```python
from build123d import *

# Parameters (mm, degrees)
PAD_DEPTH    = 1.56
PAD001_DEPTH = 1.56
SKETCH002_W  = 11.4
SKETCH002_H  = 3.36
PAD002_DEPTH = 0.1
SKETCH003_W  = 11.4
SKETCH003_H  = 0.1
PAD003_DEPTH = 9.6
FILLET_R     = 1
FILLET001_R  = 1
POCKET_DEPTH = 0.2


with BuildPart() as part:
    # Sketch → Pad (new body)
    with BuildSketch(Plane.XY):
        with BuildLine():
            Line((-9.985, 17.165), (9.985, 17.165))
            ThreePointArc((13.985, 13.165), (12.813427, 15.993427), (9.985, 17.165))
            Line((13.985, 13.165), (13.985, -13.165))
            ThreePointArc((9.985, -17.165), (12.813427, -15.993427), (13.985, -13.165))
            Line((9.985, -17.165), (-9.985, -17.165))
            ThreePointArc((-13.985, -13.165), (-12.813427, -15.993427), (-9.985, -17.165))
            Line((-13.985, -13.165), (-13.985, 13.165))
            ThreePointArc((-9.985, 17.165), (-12.813427, 15.993427), (-13.985, 13.165))
        make_face()
    extrude(amount=PAD_DEPTH)

    # Sketch001 (on Face10 of Pad) → Pad001 (join)
    with BuildSketch(Plane.XY.offset(1.56)):
        with BuildLine():
            Line((-10.035, 18.165), (10.035, 18.165))
            ThreePointArc((15.035, 13.165), (13.570534, 16.700534), (10.035, 18.165))
            Line((15.035, 13.165), (15.035, -14.264405))
            ThreePointArc((10.035, -19.264405), (13.570534, -17.799939), (15.035, -14.264405))
            Line((10.035, -19.264405), (-10.035, -19.264405))
            ThreePointArc((-15.035, -14.264405), (-13.570534, -17.799939), (-10.035, -19.264405))
            Line((-15.035, -14.264405), (-15.035, 13.165))
            ThreePointArc((-10.035, 18.165), (-13.570534, 16.700534), (-15.035, 13.165))
        make_face()
    extrude(amount=-PAD001_DEPTH)

    # Sketch002 (on Face10 of Pad001) → Pad002 (join)
    with BuildSketch(Plane.XZ.offset(19.264405)):
        with Locations((0, 1.68)):
            Rectangle(SKETCH002_W, SKETCH002_H)
    extrude(amount=PAD002_DEPTH)

    # Sketch003 (on Face11 of Pad002) → Pad003 (join)
    with BuildSketch(Plane(origin=(0, -19.264405, 0), x_dir=(-1, 0, 0), z_dir=(0, 1, 0))):
        with Locations((0, 3.31)):
            Rectangle(SKETCH003_W, SKETCH003_H)
    extrude(amount=PAD003_DEPTH)

    # Fillet
    fillet_edges = [part.edges().sort_by_distance(p)[0] for p in [
        (-5.7, -9.664405, 3.31),
    ]]
    fillet(fillet_edges, radius=FILLET_R)

    # Fillet001
    fillet001_edges = [part.edges().sort_by_distance(p)[0] for p in [
        (5.7, -9.664405, 3.31),
    ]]
    fillet(fillet001_edges, radius=FILLET001_R)

    # Sketch004 (on Face25 of Fillet001) → Pocket (cut)
    with BuildSketch(Plane(origin=(0, 0, 0), x_dir=(1, 0, 0), z_dir=(0, 0, -1))):
        with BuildLine():
            ThreePointArc((-7.5, 18.464405), (-7.75, 18.214405), (-7.5, 17.964405))
            Line((-7.5, 17.964405), (7.5, 17.964405))
            ThreePointArc((7.5, 17.964405), (7.75, 18.214405), (7.5, 18.464405))
            Line((7.5, 18.464405), (-7.5, 18.464405))
        make_face()
    extrude(amount=-POCKET_DEPTH, mode=Mode.SUBTRACT)


solid = part.part
```
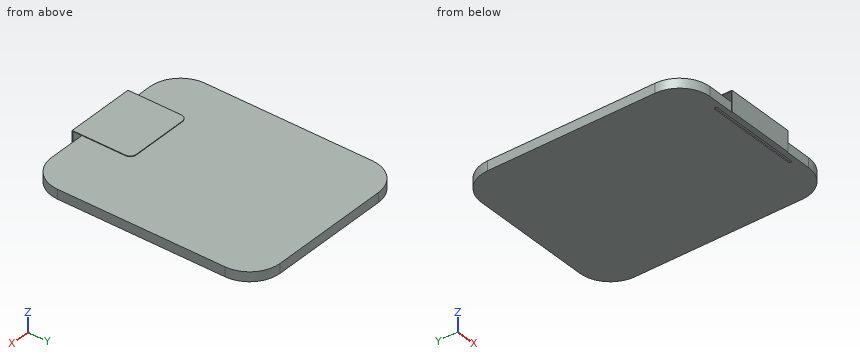
Verification items for the finished model (mm, model axes). Coordinates: 2 decimals unless noted, no trailing zeros. Order: outer loops, then holes, each group sorted by start corner. A loop starts at its lowest first (then second) coordinate and runs counter-clockwise, first axis right, second up. Notation, with made-up numbers: (24, 8.25) -> (43, 8.25) arc R30 cw to (43, 41.25) -> close; hole circle Ø5 at (80, 14). An arc over 180 degrees is marked (long way). Put each result on its own line as item: value. Start each with the question number.
1) Go/stop test with flat-tipped pins: pin 1 (2 mm diameter, centred on x = -11.5, z = 1.5, fed in from +Y); pin 2 (10.5 mm diameter, centred on x = 0.5, y = -15.5, fed in from -Z); pin 3 (1.7 mm diameter, centred on x = 8.5, z = 1, fed in from -Y); pin 4 (3 mm diameter, centred on x = 6.5, y = 0.5, fed in from +Z). Record where each tip stops, or that it passes through.
2) Material ranges on L1, parallel to Z at x = 9, y = -7; L2, parallel to X at y = -14.5, z = 0.45; L3, parallel to Y at x = 6, z = 0.85 (3 decimals), recorded low to high.
3) Cross-section at C-C (y = -0.5). Enter the section's corners in (x, z) (3 decimals).
4) Cross-section at D-D (x = 9). Enter the section's corners in (y, z) (3 decimals), plus the area to 3 significant figures.
5) Cross-section at B-B (z = 0.6). Enter the section's corners in (x, y) (3 decimals).
6) Cross-section at A-A (x = 0). Enter the section's corners in (y, z) (3 decimals), plus the area to 3 significant figures.
Geometry check:
1. pin 1: stops at y = 18.14
1. pin 2: stops at z = 0
1. pin 3: stops at y = -19.26
1. pin 4: stops at z = 1.56
2. L1: z = 0 to 1.56
2. L2: x = -15.03 to 15.03
2. L3: y = -19.264 to 18.165
3. outline: (-15.035, 0) -> (15.035, 0) -> (15.035, 1.56) -> (-15.035, 1.56) -> close
4. outline: (-19.264, 0) -> (18.165, 0) -> (18.165, 1.56) -> (-19.264, 1.56) -> close
4. area: 58.4 mm^2
5. outline: (-15.035, -14.264) arc R5 ccw to (-10.035, -19.264) -> (-5.7, -19.264) -> (-5.7, -19.364) -> (5.7, -19.364) -> (5.7, -19.264) -> (10.035, -19.264) arc R5 ccw to (15.035, -14.264) -> (15.035, 13.165) arc R5 ccw to (10.035, 18.165) -> (-10.035, 18.165) arc R5 ccw to (-15.035, 13.165) -> close
6. outline: (-19.364, 0) -> (-18.464, 0) -> (-18.464, 0.2) -> (-17.964, 0.2) -> (-17.964, 0) -> (18.165, 0) -> (18.165, 1.56) -> (-19.264, 1.56) -> (-19.264, 3.26) -> (-9.664, 3.26) -> (-9.664, 3.36) -> (-19.364, 3.36) -> close
6. area: 59.6 mm^2
